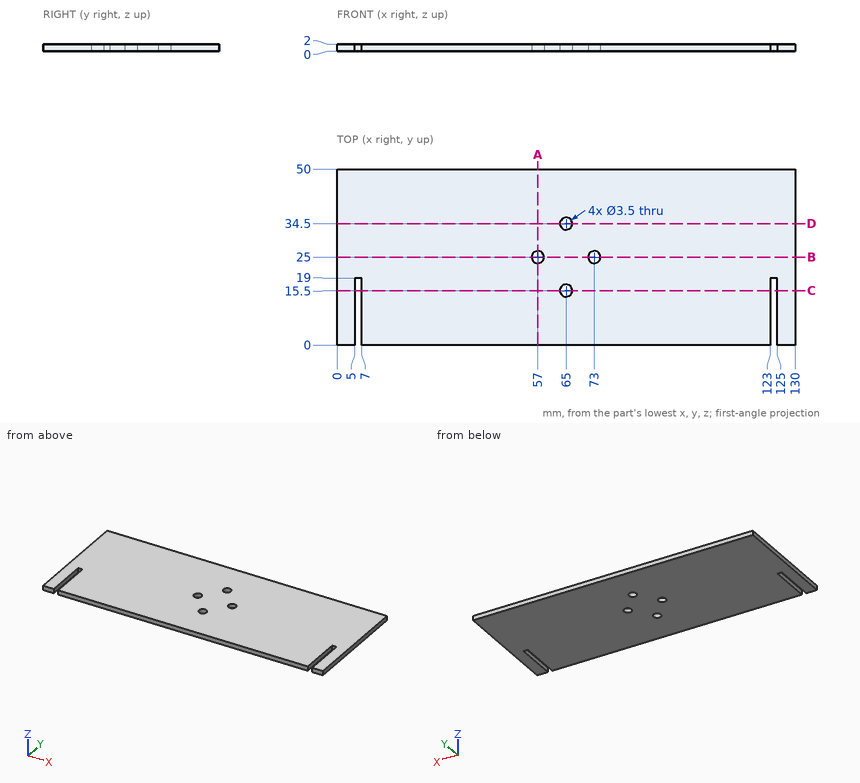
Geometry: see drawing. Coordinates: mm, zero at the bounding-box minimum. Round coordinates to 2 decimals unless told otherwise and drop trailing zeros. Write each loop counter-clockwise with the first axis right and the second up, starting at its lowest first coordinate (ties: lowest second). Pieces come first, ordered by that corner, then holes. Notation, with made-up numbers: M 26,-11 L 43,-11 A37 cw 43,25 Z; hole C -35,-1 d7. An arc over 180 degrees is marked long. Answer in a Markdown table with one row per item. Add a question column.
(1) Cut plane B-B, the plane y = 25. Return the cut outline in (x, z).
(2) Cut plane C-C, the plane y = 15.5. Return the cut outline in (x, z), then the cut area to 3 significant figures.
(3) Contact query for a flat-ended pin moving along its axis: pin 1 (1 mm diameter, centred on y = 8.5, z = 1.5, fed in from -X). Output: stop coordinate, or through.
(4) Cut plane A-A, the plane x = 57. Return the cut outline in (y, z).
(5) Cut plane D-D, the plane y = 34.5. Return the cut outline in (x, z), then the cut area to 3 significant figures.
(6) Ray query, L1, parallel to Y at x = 65, z = 0.65; L2, parallel to X at y = 8, z = 1.45; L3, parallel to Y at x = 57, z = 0.75. Return the intervals inside material, ascending.
Established:
| question | item | result |
|---|---|---|
| 1 | outline | M 0,0 L 55.25,0 L 55.25,2 L 0,2 Z; M 58.75,0 L 71.25,0 L 71.25,2 L 58.75,2 Z; M 74.75,0 L 130,0 L 130,2 L 74.75,2 Z |
| 2 | outline | M 0,0 L 5,0 L 5,2 L 0,2 Z; M 7,0 L 63.25,0 L 63.25,2 L 7,2 Z; M 66.75,0 L 123,0 L 123,2 L 66.75,2 Z; M 125,0 L 130,0 L 130,2 L 125,2 Z |
| 2 | area | 245 mm² |
| 3 | pin 1 | x = 0 |
| 4 | outline | M 0,0 L 23.25,0 L 23.25,2 L 0,2 Z; M 26.75,0 L 50,0 L 50,2 L 26.75,2 Z |
| 5 | outline | M 0,0 L 63.25,0 L 63.25,2 L 0,2 Z; M 66.75,0 L 130,0 L 130,2 L 66.75,2 Z |
| 5 | area | 253 mm² |
| 6 | L1 | 0 to 13.75, 17.25 to 32.75, 36.25 to 50 |
| 6 | L2 | 0 to 5, 7 to 123, 125 to 130 |
| 6 | L3 | 0 to 23.25, 26.75 to 50 |
